Can you work these out from the model? Positions are in its coordinate system, mm. A direction names the side the tool comes from. Round coordinates to 2 decimals unless told otherwise and drop trailing zeros. Loops run counter-clockwise (first coordinate to the right, second up) from the corner with the lowest first, then second, coordinate; pieces in that order, holes last. Notation, with made-up numbers: (29.5, -39.5) -> (70.5, -39.5) arc R16 cw to (70.5, -13.5) -> close; hole circle Ø11 at (-37.5, -30). An arc over 180 degrees is marked (long way). Write item = value, one per line.
from build123d import *

# Parameters (mm, degrees)
SKETCH1_R           = 3.175
BOSS_EXTRUDE1_DEPTH = 4
BOSS_EXTRUDE2_DEPTH = 8
BOSS_EXTRUDE3_DEPTH = 5.05
BOSS_EXTRUDE4_DEPTH = 2
BOSS_EXTRUDE5_DEPTH = 4


with BuildPart() as part:
    # Sketch1 → Boss-Extrude1 (new body)
    with BuildSketch(Plane(origin=(0, 0, 0), x_dir=(1, 0, 0), z_dir=(0, 1, 0))):
        Polygon((-11, -11), (-1, -11), (-1, 1), (11, 1), (11, 11), (-0.85301769, 11), (-8.02801769, 18.175), (-13.97198231, 18.175), (-18.175, 13.97198231), (-18.175, 8.02801769), (-11, 0.85301769), align=None)
        with Locations(Location((-11, 11, 0), (0, 0, 270))):
            Circle(SKETCH1_R, mode=Mode.SUBTRACT)
    extrude(amount=-BOSS_EXTRUDE1_DEPTH)

    # Sketch2 → Boss-Extrude2 (add)
    with BuildSketch(Plane.XZ.offset(4)):
        Polygon((-0.85301769, -11), (11, -11), (11, -5), (5.14698231, -5), align=None)
        Polygon((-11, -0.85301769), (-11, 11), (-5, 11), (-5, 5.14698231), align=None)
    extrude(amount=BOSS_EXTRUDE2_DEPTH)

    # Sketch3 → Boss-Extrude3 (add)
    with BuildSketch(Plane.XZ.offset(12)):
        Polygon((-0.85301769, -11), (11, -11), (11, -5), (5.14698231, -5), (1.632263684, -5), (-5, 1.632263684), (-5, 5.14698231), (-5, 11), (-11, 11), (-11, -0.85301769), align=None)
    extrude(amount=BOSS_EXTRUDE3_DEPTH)

    # Sketch4 → Boss-Extrude4 (add)
    with BuildSketch(Plane.XZ.offset(17.05)):
        Polygon((-5, 11), (-11, 11), (-11, -0.85301769), (-0.85301769, -11), (11, -11), (11, -5), align=None)
    extrude(amount=BOSS_EXTRUDE4_DEPTH)

    # Sketch5 → Boss-Extrude5 (add)
    with BuildSketch(Plane.XZ.offset(19.05)):
        Polygon((-19.75493597, 5.073491155), (5.073491155, -19.75493597), (16.828427125, -8), (-8, 16.828427125), align=None)
    extrude(amount=BOSS_EXTRUDE5_DEPTH)


solid = part.part
1. Suppose I cut it at A-A, the plane y = -4.75. List the corners of the cut face in (x, z) for me.
Entries:
outline = (-11, -0.85) -> (-5, 5.15) -> (-5, 11) -> (-11, 11) -> close; (-0.85, -11) -> (11, -11) -> (11, -5) -> (5.15, -5) -> close
2. For faces 1 (the flat face through (11, -7, -7)), 2 (the flat face through (-7.51, -21.02, -7.17)), 3 (the flat face through (-7.958, -7.944, 2.189)), which set-ups out of +Z, -Z, +X, -X, +Y, -Y let a thin tool reach every point of the face, with its end or its side?
Entries:
face_1 = +Z, -Z, +X, +Y
face_2 = -Z, -X, -Y
face_3 = -Z, +X
3. Suppose I cut it at B-B, the plane z = -3. List the corners of the cut face in (x, y) for me.
Entries:
outline = (-13.15, -4) -> (11, -4) -> (11, 0) -> (-13.15, 0) -> close; (-11.68, -23.05) -> (11.83, -23.05) -> (11.83, -19.05) -> (9, -19.05) -> (9, -17.05) -> (-0.37, -17.05) -> (-0.37, -12) -> (-8.85, -12) -> (-8.85, -19.05) -> (-11.68, -19.05) -> close
4. I'm going to push flat-ended pins straight in: pin 1 (3 mm diameter, centred on x = -9.5, y = -2.5, fed in from -Z) (3 decimals); pin 2 (3 mm diameter, centred on x = 3, y = -1.5, fed in from +Z); pin 3 (2 mm diameter, centred on y = -2, z = 3, fed in from +X); pin 4 (11 mm diameter, centred on x = -7.5, z = -5, fed in from +Y). Where does each tip first touch, or does it pass through?
Entries:
pin_1 = -18.175
pin_2 = -1
pin_3 = -1
pin_4 = 0
5. Suppose I cut it at D-D, the plane y = -13.75. List the corners of the cut face in (x, z) for me, and give its area (3 significant figures).
Entries:
outline = (-11, -0.85) -> (-0.85, -11) -> (11, -11) -> (11, -5) -> (1.63, -5) -> (-5, 1.63) -> (-5, 11) -> (-11, 11) -> close
area = 199 mm²
6. Suppose I cut it at C-C, the plane x = -2. List the corners of the cut face in (y, z) for me.
Entries:
outline = (-23.05, -12.68) -> (-19.05, -12.68) -> (-19.05, -9.85) -> (-12, -9.85) -> (-12, -1.37) -> (-17.05, -1.37) -> (-17.05, 8) -> (-19.05, 8) -> (-19.05, 10.83) -> (-23.05, 10.83) -> close; (-4, -12.15) -> (0, -12.15) -> (0, 11) -> (-4, 11) -> close
7. We'd pull the mould along Z, two halves only. Please class faces 4 (the flat face through (-1.64, -14.49, -1.73)), 5 (the cylindrical face through (-13.8, -2, -9.5)), 6 (the flat face through (-7, -4, -7)): released by +Z, released by -Z, zero draft, split by the parting line, or undercut.
Entries:
face_4 = released by +Z
face_5 = undercut
face_6 = zero draft
8. I need wall thicknesses on line 1 (X direction, y = -3.5, z = -12.5) (3 decimals); line 2 (Y direction, x = -5.5, z = -11); line 3 (Y direction, x = -4, z = 1). Which ranges of each line are inside material? Lowest first, please. Write a range as [from, to].
Entries:
line_1 = [-18.175, -13.798], [-8.202, -2.353]
line_2 = [-4, 0]
line_3 = [-23.05, -17.05], [-4, 0]
